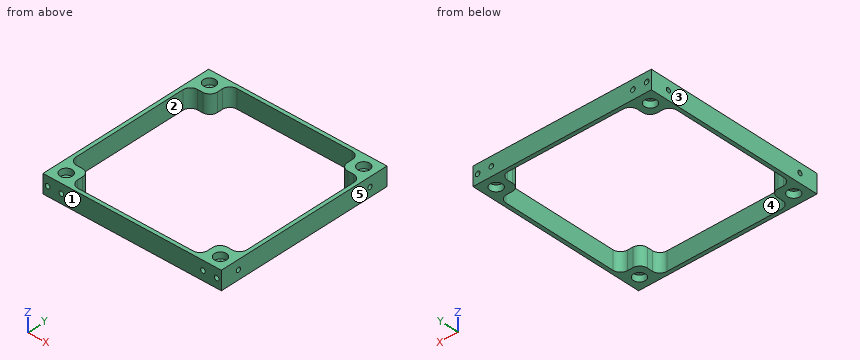
from build123d import *

# Parameters (mm, degrees)
BOTTOMLAYER_DEPTH                                   = 10
CBORE_FOR_M3_HEX_SOCKET_HEAD_CAP_SCREW1_D           = 3.4
CBORE_FOR_M3_HEX_SOCKET_HEAD_CAP_SCREW1_CBORE_D     = 6.5
CBORE_FOR_M3_HEX_SOCKET_HEAD_CAP_SCREW1_CBORE_DEPTH = 3.4
CIRPATTERN1_COUNT                                   = 4
CUT_EXTRUDE1_START                                  = -3.4
SKETCH30_R                                          = 3.25
CUT_EXTRUDE1_DEPTH                                  = 3.4
CIRPATTERN2_COUNT                                   = 4


with BuildPart() as part:
    # Sketch3 → BottomLayer (new body)
    with BuildSketch(Plane.XY):
        with BuildLine():
            Line((0, 48), (48, 48))
            Line((48, 48), (48, 0))
            Line((48, 0), (46, 0))
            Line((46, 0), (46, 31))
            ThreePointArc((46, 31), (44.828427125, 33.828427125), (42, 35))
            Line((42, 35), (39, 35))
            ThreePointArc((39, 35), (36.171572875, 36.171572875), (35, 39))
            Line((35, 39), (35, 42))
            ThreePointArc((35, 42), (33.828427125, 44.828427125), (31, 46))
            Line((31, 46), (0, 46))
            Line((0, 46), (0, 48))
        make_face()
    bottomlayer = extrude(amount=BOTTOMLAYER_DEPTH)

    # CBORE for M3 Hex Socket Head Cap Screw1 (through all)
    with Locations(Plane.XY.offset(10)):
        with Locations((41.525, 41.525)):
            cbore_for_m3_hex_socket_head_cap_screw1 = CounterBoreHole(CBORE_FOR_M3_HEX_SOCKET_HEAD_CAP_SCREW1_D / 2, CBORE_FOR_M3_HEX_SOCKET_HEAD_CAP_SCREW1_CBORE_D / 2, CBORE_FOR_M3_HEX_SOCKET_HEAD_CAP_SCREW1_CBORE_DEPTH)

    # CirPattern1: BottomLayer, CBORE for M3 Hex Socket Head Cap Screw1 ×4 about axis
    cirpattern1_axis = Axis((0, 0, 0), (0, 0, 1))
    add([bottomlayer.rotate(cirpattern1_axis, i * 360 / CIRPATTERN1_COUNT) for i in range(1, CIRPATTERN1_COUNT)])
    add([cbore_for_m3_hex_socket_head_cap_screw1.rotate(cirpattern1_axis, i * 360 / CIRPATTERN1_COUNT) for i in range(1, CIRPATTERN1_COUNT)], mode=Mode.SUBTRACT)

    # Sketch21 → Tap Drill M3 Side Plate (revolve, cut)
    with BuildSketch(Plane(origin=(48, 38.1, 5), x_dir=(0, 0, -1), z_dir=(0, 1, 0))):
        Polygon((0, 0), (0, 5.751075774), (1.25, 5), (1.25, 0), align=None)
    tap_drill_m3_side_plate = revolve(axis=Axis((54.35, 38.1, 5), (-1, 0, 0)), mode=Mode.SUBTRACT)

    # Sketch27 → Tap Drill M3 Side Plate 2 (revolve, cut)
    with BuildSketch(Plane(origin=(38.1, 48, 5), x_dir=(0, 0, 1), z_dir=(1, 0, 0))):
        Polygon((0, 0), (0, 5.751075774), (1.25, 5), (1.25, 0), align=None)
    tap_drill_m3_side_plate_2 = revolve(axis=Axis((38.1, 54.35, 5), (0, -1, 0)), mode=Mode.SUBTRACT)

    # Sketch29 → Tap Drill M3 Rail (revolve, cut)
    with BuildSketch(Plane(origin=(45.5, 48, 5), x_dir=(0, 0, 1), z_dir=(1, 0, 0))):
        Polygon((0, 0), (0, 5.751075774), (1.25, 5), (1.25, 0), align=None)
    tap_drill_m3_rail = revolve(axis=Axis((45.5, 54.35, 5), (0, -1, 0)), mode=Mode.SUBTRACT)

    # SidePlate and Rail Holes 1: Tap Drill M3 Side Plate, Tap Drill M3 Side Plate 2, Tap Drill M3 Rail across plane
    add(tap_drill_m3_side_plate.mirror(Plane(origin=(0, 0, 0), x_dir=(0, 0, 1), z_dir=(1, 0, 0))), mode=Mode.SUBTRACT)
    add(tap_drill_m3_side_plate_2.mirror(Plane(origin=(0, 0, 0), x_dir=(0, 0, 1), z_dir=(1, 0, 0))), mode=Mode.SUBTRACT)
    add(tap_drill_m3_rail.mirror(Plane(origin=(0, 0, 0), x_dir=(0, 0, 1), z_dir=(1, 0, 0))), mode=Mode.SUBTRACT)

    # Side Plate and Rail Holes 2: Tap Drill M3 Side Plate, Tap Drill M3 Side Plate 2, Tap Drill M3 Rail across plane
    add(tap_drill_m3_side_plate.mirror(Plane.ZX), mode=Mode.SUBTRACT)
    add(tap_drill_m3_side_plate_2.mirror(Plane.ZX), mode=Mode.SUBTRACT)
    add(tap_drill_m3_rail.mirror(Plane.ZX), mode=Mode.SUBTRACT)

    # Side Plate and Rail Holes 2 copy 1 sketc → Side Plate and Rail Holes 2 copy 1 (revolve, cut)
    with BuildSketch(Plane(origin=(-48, -38.1, 5), x_dir=(0, 0, -1), z_dir=(0, -1, 0))):
        Polygon((0, 0), (0, 5.751075774), (1.25, 5), (1.25, 0), align=None)
    revolve(axis=Axis((-54.35, -38.1, 5), (1, 0, 0)), mode=Mode.SUBTRACT)

    # Side Plate and Rail Holes 2 copy 2 sketc → Side Plate and Rail Holes 2 copy 2 (revolve, cut)
    with BuildSketch(Plane(origin=(-38.1, -48, 5), x_dir=(0, 0, 1), z_dir=(-1, 0, 0))):
        Polygon((0, 0), (0, 5.751075774), (1.25, 5), (1.25, 0), align=None)
    revolve(axis=Axis((-38.1, -54.35, 5), (0, 1, 0)), mode=Mode.SUBTRACT)

    # Side Plate and Rail Holes 2 copy 3 sketc → Side Plate and Rail Holes 2 copy 3 (revolve, cut)
    with BuildSketch(Plane(origin=(-45.5, -48, 5), x_dir=(0, 0, 1), z_dir=(-1, 0, 0))):
        Polygon((0, 0), (0, 5.751075774), (1.25, 5), (1.25, 0), align=None)
    revolve(axis=Axis((-45.5, -54.35, 5), (0, 1, 0)), mode=Mode.SUBTRACT)

    # Sketch30 → Cut-Extrude1 (cut)
    with BuildSketch(Plane(origin=(0, 0, 0), x_dir=(-1, 0, 0), z_dir=(0, 0, -1)).offset(CUT_EXTRUDE1_START)):
        with Locations(Location((-41.525, 41.525, 0), (0, 0, 180))):
            Circle(SKETCH30_R)
    cut_extrude1 = extrude(amount=CUT_EXTRUDE1_DEPTH, mode=Mode.SUBTRACT)

    # CirPattern2: Cut-Extrude1 ×4 about axis
    cirpattern2_axis = Axis((0, 0, 0), (0, 0, 1))
    for i in range(1, CIRPATTERN2_COUNT):
        add(cut_extrude1.rotate(cirpattern2_axis, i * 360 / CIRPATTERN2_COUNT), mode=Mode.SUBTRACT)


solid = part.part
Build history of the part. All positions in model axes, mm. Face numbers are marked on the shaded views. A direction names the side the tool comes from. Coordinates: 2 decimals unless noted, no trailing zeros. Order: outer loops, then holes, each group sorted by start corner. A loop starts at its lowest first (then second) coordinate and runs counter-clockwise, first axis right, second up. Notation, with made-up numbers: (11.5, -30.5) - (20.5, -30.5) arc R14 ccw to (20.5, -19.5) - close; hole circle Ø10 at (12.25, -27). An arc over 180 degrees is marked (long way). Write each question's results on one line, items separated by ' | '. Start each with the question number.
Item 1: Band-saw the part on A-A on x = -18.5. Write the cut outline in (y, z), and give its area (3 significant figures).
Item 2: Band-saw the part on C-C on z = 7.75. State how many separate pieces and enclosed holes the cut face has, and give its area (3 significant figures).
Item 3: Mould opens along Y. For the marked faces 1, 2 and 3 say: released by +Y, released by -Y, zero draft, split by the parting line, or undercut.
Item 4: Flat gauge pins, fed straight in: pin 1 (2 mm diameter, centred on x = 45.5, z = 5, fed in from -Y); pin 2 (2.5 mm diameter, centred on x = -41.525, y = 41.525, fed in from +Z); pin 3 (5 mm diameter, centred on x = 40.5, y = -41.5, fed in from +Z); pin 4 (2 mm diameter, centred on y = -38.1, z = 5, fed in from +X). Where does each tip first touch, or does it go through?
Item 5: Tool access for the marked faces 4 and 5: list every direction of +Z, -Z, +X, -X, +Y, -Y with a clear straight run to the whole face (end or side of a thin tool).
Item 6: Wall check: probe 1 along X at (y, z) = (8.5, 7); probe 2 along Y at (x, z) = (-46.55, 5). Give the ranges that are in metal, low to high. Write a range as [from, to].
Numbers:
1) outline: (-48, 0) - (-46, 0) - (-46, 10) - (-48, 10) - close; (46, 0) - (48, 0) - (48, 10) - (46, 10) - close | area: 40.0 mm^2
2) separate pieces: 1 | enclosed holes: 5 | area: 1,120 mm^2
3) face 1: released by -Y | face 2: undercut | face 3: zero draft
4) pin 1: y = -42.85 | pin 2: through | pin 3: z = 10 | pin 4: x = 42.85
5) face 4: +Z, -Z | face 5: +Z, -Z, +X, +Y, -Y
6) probe 1: [-48, -46], [46, 48] | probe 2: [-42.88, -39.35], [-36.85, 36.85], [39.35, 42.88]
